Here's how the part is built. I have some questions about the finished solid (model axes, mm). Face numbers are marked on the shaded views. Give positions to 0.01 mm unless a question says otherwise; leave off trailing zeros. Order: outer loops, then holes, each group sorted by start corner. A loop starts at its lowest first (then second) coordinate and runs counter-clockwise, first axis right, second up. Notation, with made-up numbers: (-22, 42) - (26, 42) arc R31 ccw to (26, 72) - close; hole circle Ø11 at (27, -20). An arc over 180 degrees is marked (long way). One line per question, with ' | ' between items.
from build123d import *

# Parameters (mm, degrees)
EXTRUDE_1_DEPTH       = 2
EXTRUDE_1_DEPTH_BACK  = 2
SKETCH_1_W            = 60
SKETCH_1_H            = 30
SKETCH_2_W            = 56.5
SKETCH_2_H            = 25.5
CUT_EXTRUDE_1_DEPTH   = 2.5
CHAMFER_1_SIZE        = 1
EXTRUDE_2_DEPTH       = 15
MIRROR_2_COPY_1_DEPTH = 15
FILLET_1_R            = 0.1


with BuildPart() as part:
    # 草图1 → 凸台-拉伸1 (new, two sides: drawn at the far end of the back side and taken through both)
    with BuildSketch(Plane(origin=(0, 0, 0), x_dir=(1, 0, 0), z_dir=(0, 1, 0)).offset(-EXTRUDE_1_DEPTH_BACK)):
        Rectangle(SKETCH_1_W, SKETCH_1_H)
    extrude(amount=EXTRUDE_1_DEPTH + EXTRUDE_1_DEPTH_BACK)

    # 草图2 → 切除-拉伸1 (cut)
    with BuildSketch(Plane(origin=(0, 2, 0), x_dir=(1, 0, 0), z_dir=(0, 1, 0))):
        Rectangle(SKETCH_2_W, SKETCH_2_H)
    extrude(amount=-CUT_EXTRUDE_1_DEPTH, mode=Mode.SUBTRACT)

    # 倒角1
    chamfer_1_edges = [part.edges().sort_by_distance(p)[0] for p in [
        (0, -0.5, -12.75),
        (28.25, -0.5, 0),
        (0, -0.5, 12.75),
        (-28.25, -0.5, 0),
    ]]
    chamfer(chamfer_1_edges, length=CHAMFER_1_SIZE)

    # 草图3 → 凸台-拉伸2 (add, symmetric)
    with BuildSketch(Plane.XY):
        with BuildLine():
            Line((30.677124344, 1.5), (30, 1.5))
            Line((30, 1.5), (30, 0))
            Line((30, 0), (32.5, 1.165769145))
            Line((32.5, 1.165769145), (32.5, 1.95))
            Line((32.5, 1.95), (31.555590279, 1.95))
            ThreePointArc((31.555590279, 1.95), (31.088161527, 1.780042303), (30.677124344, 1.5))
        make_face()
    extrude_2 = extrude(amount=EXTRUDE_2_DEPTH, both=True)

    # 镜向1: 凸台-拉伸2 across plane
    add(extrude_2.mirror(Plane.ZX))

    # 镜向2: 凸台-拉伸2 across plane
    add(extrude_2.mirror(Plane(origin=(0, 0, 0), x_dir=(0, 0, 1), z_dir=(1, 0, 0))))

    # 镜向2 copy 1 sketch → 镜向2 copy 1 (add, symmetric)
    with BuildSketch(Plane(origin=(0, 0, 0), x_dir=(-1, 0, 0), z_dir=(0, 0, 1))):
        with BuildLine():
            Line((30.677124344, 1.5), (30, 1.5))
            Line((30, 1.5), (30, 0))
            Line((30, 0), (32.5, 1.165769145))
            Line((32.5, 1.165769145), (32.5, 1.95))
            Line((32.5, 1.95), (31.555590279, 1.95))
            ThreePointArc((31.555590279, 1.95), (31.088161527, 1.780042303), (30.677124344, 1.5))
        make_face()
    extrude(amount=MIRROR_2_COPY_1_DEPTH, both=True)

    # 圆角1
    fillet_1_edges = [part.edges().sort_by_distance(p)[0] for p in [
        (-32.5, -1.95, 0),
        (32.5, 1.95, 0),
        (32.5, -1.95, 0),
        (-32.5, 1.95, 0),
    ]]
    fillet(fillet_1_edges, radius=FILLET_1_R)


solid = part.part
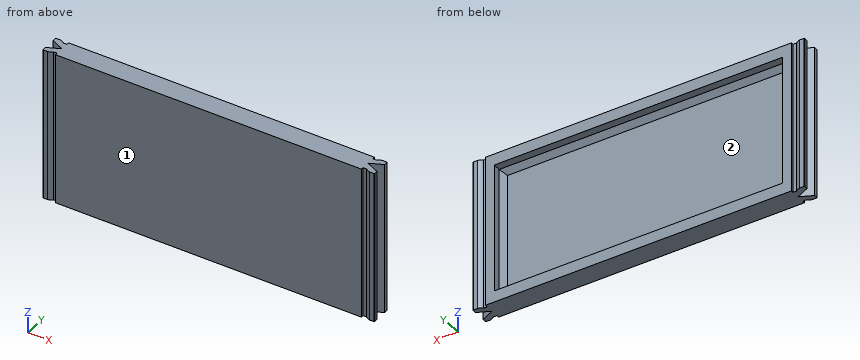
1) Please list where these lines run through material, in increasing order: L1, parallel to X at y = 1.7, z = -1; L2, parallel to Z at x = -25, y = 0.75.
Model answer:
L1: x = -32.5 to -30.95, -30 to -28.25, 28.25 to 30, 30.95 to 32.5 | L2: z = -15 to -12.75, 12.75 to 15
2) I want a section at A-A (x = 18). List the corners of the cut face in (y, z) for me.
Model answer:
outline: (-2, -15) - (2, -15) - (2, -12.75) - (0.5, -12.75) - (-0.5, -11.75) - (-0.5, 11.75) - (0.5, 12.75) - (2, 12.75) - (2, 15) - (-2, 15) - close
3) Thinking about a two-plate mould opening in Z: for the marked faces 1 and 2, which applies, +Z half, -Z half, draft (parallel to the pull), parting line (faces both ways), or undercut?
Model answer:
face 1: draft | face 2: undercut
4) I'm going to push flat-ended pins straight in: P1, Ø5, axis at x = -4, z = 8.5, coming from the +Y side; P2, Ø0.7, axis at x = -30.5, z = -0.5, coming from the +Y side; P3, Ø0.5, axis at x = 30.5, z = -1, coming from the -Y side. Where does each tip first touch, or does it pass through?
Model answer:
P1: stops at y = -0.5 | P2: stops at y = 1.64 | P3: stops at y = -1.56
